Geometry: final body of the model. Coordinates: model frame, mm. A direction names the side the tool comes from. Round coordinates to 2 decimals unless told otherwise and drop trailing zeros. Loops run counter-clockwise (first coordinate to the right, second up) from the corner with the lowest first, then second, coordinate; pieces in that order, holes last. Notation, with made-up numbers: M -26.5,23 L -9.5,23 A14 cw -9.5,38 Z; hole C 67,88 d9. An arc over 180 degrees is marked long. Write each question's results on one line, items separated by ' | '.
```python
from build123d import *

# Parameters (mm, degrees)
BOSS_EXTRUDE1_DEPTH = 12
FILLET1_R           = 1
SKETCH4_R           = 2
CUT_EXTRUDE1_DEPTH  = 16.81929202
THREAD1_PITCH       = 0.7
CHAMFER2_SIZE       = 0.5
CHAMFER4_SIZE       = 0.5
CUT_EXTRUDE2_DEPTH  = 0.3
FILLET4_R           = 0.25


with BuildPart() as part:
    # Sketch2 → Boss-Extrude1 (new body)
    with BuildSketch(Plane(origin=(0, 0, 0), x_dir=(1, 0, 0), z_dir=(0, 1, 0))):
        Polygon((0, 0), (8, 0), (9.5, 2), (9.5, 3.25), (9.25, 3.25), (9.25, 3), (7.25, 3), (7.25, 4), (5.25, 4), (4, 3.5), (2.75, 4), (0.75, 4), (0.75, 3), (-1.25, 3), (-1.25, 3.25), (-1.5, 3.25), (-1.5, 2), align=None)
    extrude(amount=BOSS_EXTRUDE1_DEPTH)

    # Fillet1
    fillet1_edges = [part.edges().sort_by_distance(p)[0] for p in [
        (-1.5, 6, -2),
        (9.5, 6, -2),
        (8, 6, 0),
        (0, 6, 0),
    ]]
    fillet(fillet1_edges, radius=FILLET1_R)

    # Sketch4 → Cut-Extrude1 (cut, through all)
    with BuildSketch(Plane(origin=(0, 0, -4), x_dir=(-1, 0, 0), z_dir=(0, 0, -1))):
        with Locations((-4, 6)):
            Circle(SKETCH4_R)
    extrude(amount=-CUT_EXTRUDE1_DEPTH, mode=Mode.SUBTRACT)

    # Thread1: arcs per turn and ends read off the stored shape
    # Thread1: the profile of Thread Profile1 profile screwed along a right-hand helix through 3.285711 turns, 6 arcs to a turn; built about Z, then put on its axis
    thread1_z = Axis((0, 0, 0), (0, 0, 1))
    thread1_corners = [(2.0003, 0, -0.000173205), (2.0003, 0, 0.612673203), (1.621113887, 0, 0.393749999), (1.621113887, 0, 0.218749999)]
    with BuildLine(mode=Mode.PRIVATE) as thread1_profile:
        Line(thread1_corners[0], thread1_corners[1])
        Line(thread1_corners[1], thread1_corners[2])
        Line(thread1_corners[2], thread1_corners[3])
        Line(thread1_corners[3], thread1_corners[0])
    thread1_cap = Face(thread1_profile.wire())
    thread1_turn_angles = [0, 30, 60, 90, 120, 150, 180, 210, 240, 270, 300, 330, 360]
    thread1_turn_weights = [1, 0.8660254037844387, 1, 0.8660254037844387, 1, 0.8660254037844387, 1, 0.8660254037844387, 1, 0.8660254037844387, 1, 0.8660254037844387, 1]
    thread1_turn_rails = [Edge.make_bspline([Vector(p[0], p[1], 0).rotate(thread1_z, thread1_turn_angles[k]) / thread1_turn_weights[k] + Vector(0, 0, p[2] + THREAD1_PITCH * thread1_turn_angles[k] / 360) for k in range(13)], [0, 0, 0, 1, 1, 2, 2, 3, 3, 4, 4, 5, 5, 6, 6, 6], 2, thread1_turn_weights) for p in thread1_corners]
    thread1_turn_sides = [Face.make_surface_from_curves(thread1_turn_rails[p[0]], thread1_turn_rails[p[1]]) for p in [(0, 1), (1, 2), (2, 3), (3, 0)]]
    thread1_last_angles = [1080, 1110, 1140, 1161.428, 1182.856]
    thread1_last_weights = [1, 0.8660254037844387, 1, 0.9308773922572046, 1]
    thread1_last_rails = [Edge.make_bspline([Vector(p[0], p[1], 0).rotate(thread1_z, thread1_last_angles[k]) / thread1_last_weights[k] + Vector(0, 0, p[2] + THREAD1_PITCH * thread1_last_angles[k] / 360) for k in range(5)], [0, 0, 0, 1, 1, 2, 2, 2], 2, thread1_last_weights) for p in thread1_corners]
    thread1_last_sides = [Face.make_surface_from_curves(thread1_last_rails[p[0]], thread1_last_rails[p[1]]) for p in [(0, 1), (1, 2), (2, 3), (3, 0)]]
    thread1 = Plane(origin=(4, 6, -3.5), x_dir=(1, 0, 0), z_dir=(0, 0, 1)) * Solid(Shell([*[p.moved(Location((0, 0, THREAD1_PITCH * i))) for i in range(3) for p in thread1_turn_sides], *thread1_last_sides, thread1_cap, thread1_cap.rotate(thread1_z, 1182.856).moved(Location((0, 0, THREAD1_PITCH * 1182.856 / 360)))]))
    add(thread1)

    # Chamfer2
    # the kernel refuses this chamfer: 0.5 mm, written as the material it takes off along each edge
    with BuildSketch(Plane(origin=(4, 6, -4), x_dir=(-0.4063033524336664, 0.9137382479688392, 0), z_dir=(-0.9137382479688392, -0.4063033524336664, 0))) as chamfer2_piece_1:
        Polygon((2 + CHAMFER2_SIZE, 0), (2, -CHAMFER2_SIZE), (2, 0), align=None)
    revolve(axis=Axis((4, 6, -4), (0, 0, -1)), revolution_arc=227.945655457, mode=Mode.SUBTRACT)
    with BuildSketch(Plane(origin=(4, 6, -4), x_dir=(-1, 0, 0), z_dir=(0, -1, 0))) as chamfer2_piece_2:
        Polygon((2 + CHAMFER2_SIZE, 0), (2, -CHAMFER2_SIZE), (2, 0), align=None)
    revolve(axis=Axis((4, 6, -4), (0, 0, -1)), revolution_arc=113.948286938, mode=Mode.SUBTRACT)
    with BuildSketch(Plane(origin=(4, 6, -4), x_dir=(0.4059119450129516, -0.9139121910204517, 0), z_dir=(0.9139121910204517, 0.4059119450129516, 0))) as chamfer2_piece_3:
        Polygon((2 + CHAMFER2_SIZE, 0), (2, -CHAMFER2_SIZE), (2, 0), align=None)
    revolve(axis=Axis((4, 6, -4), (0, 0, -1)), revolution_arc=113.948286938, mode=Mode.SUBTRACT)

    # Chamfer4
    chamfer4_edges = [part.edges().sort_by_distance(p)[0] for p in [
        (6, 6, 0),
    ]]
    chamfer(chamfer4_edges, length=CHAMFER4_SIZE)

    # Sketch8 → Cut-Extrude2 (cut)
    with BuildSketch(Plane(origin=(0, 0, -3.25), x_dir=(-1, 0, 0), z_dir=(0, 0, -1))):
        with BuildLine():
            Line((-9.5, 10), (-9.5, 2))
            ThreePointArc((-9.5, 2), (-7.774917218, 6), (-9.5, 10))
        make_face()
        with BuildLine():
            Line((1.5, 10), (1.5, 2))
            ThreePointArc((1.5, 2), (-0.225082782, 6), (1.5, 10))
        make_face()
    extrude(amount=-CUT_EXTRUDE2_DEPTH, mode=Mode.SUBTRACT)

    # Fillet4
    fillet4_edges = [part.edges().sort_by_distance(p)[0] for p in [
        (-1.5, 11, -3.25),
        (-1.5, 1, -3.25),
        (9.5, 11, -3.25),
        (9.5, 1, -3.25),
    ]]
    fillet(fillet4_edges, radius=FILLET4_R - 0.0001)  # a hair under: the kernel refuses the full size


solid = part.part
```
1. Ray query, probe 1 along X at (y, z) = (6, -2.85); probe 2 along Y at (x, z) = (4, -0.85); probe 3 along Y at (x, z) = (4, -3.3). Return the intervals inside material, ascending.
Answer key:
probe 1: x = -1.5 to 2.38, 6 to 9.5 | probe 2: y = 0 to 4, 7.62 to 12 | probe 3: y = 0 to 4, 7.96 to 12
2. Access query for faces 4 (the face through (0.4, 5.9, -3)), 5 (the face through (9, 6, -2.95)), 6 (the face through (-1, 6, -2.95)), 7 (the face through (6.135, 6.047, -3.635)). Directions: +Z, -Z, +X, -X, +Y, -Y. A direction counts if a zero-diameter tool reaches every point of the face in a straight line with its end or side. Return the directions, or none.
Answer key:
face 4: -Z, +Y, -Y | face 5: -Z, +X | face 6: -Z, -X | face 7: -Z
3. Draft query along Z for faces 1 (the face through (4.63, 9.97, -3.75)), 2 (the face through (-0.81, 5.92, -1.08)), 3 (the face through (7.25, 5.9, -3.5)). Return one class per face: pulls with the +Z half, pulls with the -Z half, needs draft (parallel to the pull), parting line crosses it, or undercut.
Answer key:
face 1: pulls with the -Z half | face 2: pulls with the +Z half | face 3: needs draft
4. Section A-A (x = 8.5). Output: boundary loops of the cut face in (y, z).
Answer key:
outline: M 0,-3 L 3.27,-3 L 3.27,-2.95 L 8.73,-2.95 L 8.73,-3 L 12,-3 L 12,-0.67 L 0,-0.67 Z
5. Pin query (flat end, axial travel): P1, Ø6.5, axis at x = 4, y = 6, coming from the -Z side; P2, Ø0.8, axis at y = 8.5, z = -3.5, coming from the -X side; P3, Ø2, axis at x = 8.5, y = 5.5, coming from the -Z side. Return the tip coordinate at first contact, or that it passes through.
Answer key:
P1: stops at z = -4 | P2: stops at x = 0.75 | P3: stops at z = -3
